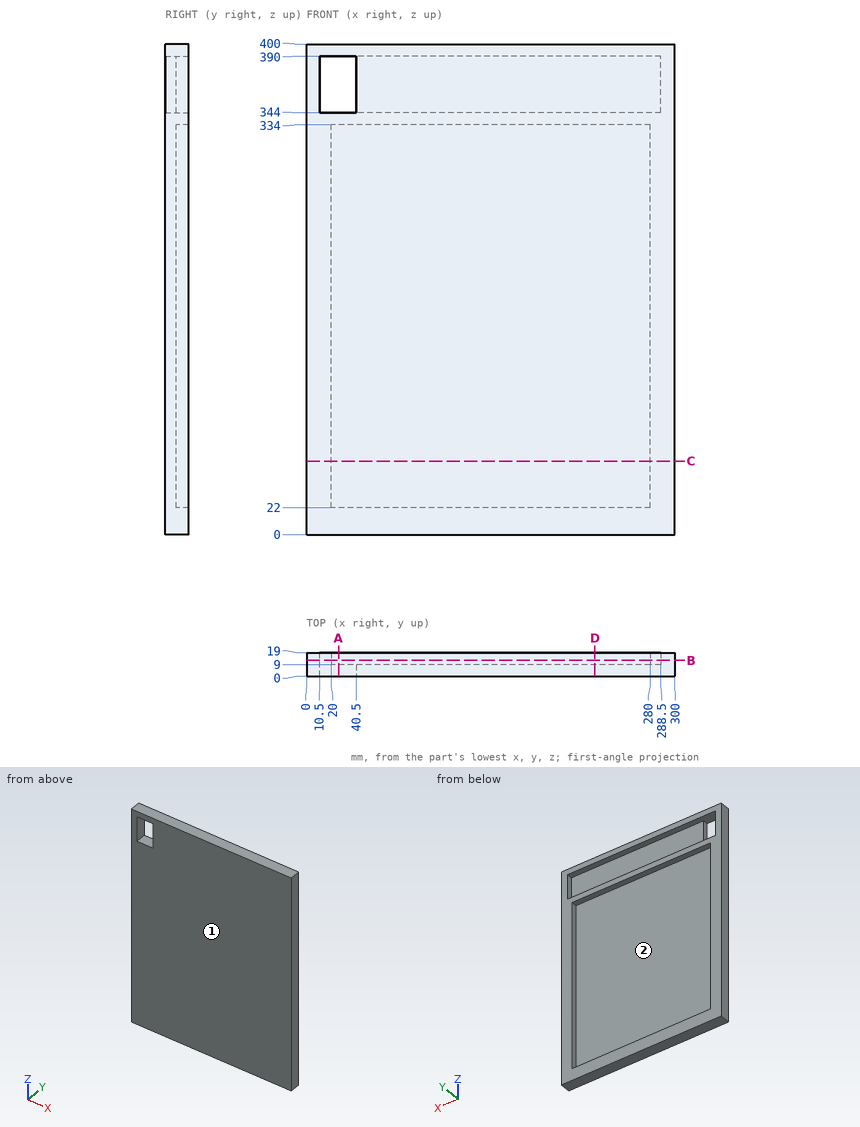
Here's the drawing with two shaded views (mm, measured from the low corner). I have some questions. Coordinates: 2 decimals unless noted, no trailing zeros. Write each loop counter-clockwise with the first axis right and the second up, starting at its lowest first coordinate (ties: lowest second). Pieces come first, ordered by that corner, then holes.
Item 1: I want a section at C-C on z = 60. Write out the boundary of the cut face in (x, y).
Item 2: I want a section at A-A on x = 26. Write out the boundary of the cut face in (y, z).
Item 3: If we mould it in two halves opening along X, with no side actions, what happens to the marked faces 1 and 2? For each: +X half, -X half, draft (parallel to the pull), parting line (faces both ways), or undercut.
Item 4: I want a section at D-D on x = 235. Write out the boundary of the cut face in (y, z), and give its area (3 significant figures).
Item 5: Will this pin go through, and if not, where does the flat tip stop? pin 1 (14 mm diameter, centred on x = 212, z = 356.5, fed in from +Y).
Item 6: If I drill on line 1 (Z direction, x = 29, y = 9.5); line 2 (X direction, y = 10.5, z = 64); line 3 (Z direction, x = 27, y = 7.5), over which ranges is the centre line in solid material (lowest first)?
Item 7: I want a section at B-B on y = 12.75. Write out the boundary of the cut face in (x, z), and give its area (3 significant figures).
Findings below:
1. outline: (0, 0) - (300, 0) - (300, 19) - (280, 19) - (280, 9) - (20, 9) - (20, 19) - (0, 19) - close
2. outline: (0, 0) - (19, 0) - (19, 22) - (9, 22) - (9, 334) - (19, 334) - (19, 344) - (0, 344) - close; (0, 390) - (19, 390) - (19, 400) - (0, 400) - close
3. face 1: draft
3. face 2: undercut
4. outline: (0, 0) - (19, 0) - (19, 22) - (9, 22) - (9, 334) - (19, 334) - (19, 344) - (9, 344) - (9, 390) - (19, 390) - (19, 400) - (0, 400) - close
4. area: 4,020 mm2
5. pin 1: stops at y = 9
6. line 1: z = 0 to 22, 334 to 344, 390 to 400
6. line 2: x = 0 to 20, 280 to 300
6. line 3: z = 0 to 344, 390 to 400
7. outline: (0, 0) - (300, 0) - (300, 400) - (0, 400) - close; hole (10.5, 344) - (288.5, 344) - (288.5, 390) - (10.5, 390) - close; hole (20, 22) - (280, 22) - (280, 334) - (20, 334) - close
7. area: 26,100 mm2
